Solid Edge part; units mm, degrees
sketch "Sketch1" plane through (0, 0, 0) normal (0, -1, 0) x (1, 0, 0)
  line L0 (40, 40) -> (-40, 40)
  line L1 (-40, 40) -> (-40, -40)
  line L2 (-40, -40) -> (40, -40)
  line L3 (40, -40) -> (40, 40)
  circle A0 centre (0, 0) radius 24
extrude "Extrusionsausprägung_23" add sketch "Sketch1" against normal blind 10
hole "Bohrung_5" at (0, 0, 30) direction (0, 1, 0) diameter 5.5 end up to next
hole "Hole1" at (30, 0, 0) direction (0, 1, 0) diameter 5.5 end up to next
hole "Hole2" at (0, 0, -30) direction (0, 1, 0) diameter 5.5 end up to next
hole "Hole3" at (-30, 0, 0) direction (0, 1, 0) diameter 5.5 end up to next
sketch "Sketch2" plane through (0, 0, 0) normal (0, -1, 0) x (1, 0, 0)
  circle A0 centre (-30, 30) radius 6.35
  circle A1 centre (30, 30) radius 6.35
  circle A2 centre (30, -30) radius 6.35
  circle A3 centre (-30, -30) radius 6.35
extrude "Extrusionsausschnitt_26" cut sketch "Sketch2" against normal blind 274
Design review of the part built by this model. Coordinates are the model's own, in mm. Round coordinates to 2 decimals unless told otherwise and drop trailing zeros. Order: outer loops, then holes, each group sorted by start corner. A loop starts at its lowest first (then second) coordinate and runs counter-clockwise, first axis right, second up. Notation, with made-up numbers: (-21.5, 2) - (21.5, 2) arc R17 ccw to (21.5, 9) - close; hole circle Ø10 at (21, -23.75). An arc over 180 degrees is marked (long way). One line per question, with ' | ' between items.
Item 1: Take a section at C-C, the plane y = 3.25. Give the number of separate pieces and of enclosed holes in the cut face, then the cut area to 3 significant figures.
Checks:
separate pieces: 1 | enclosed holes: 9 | area: 3,990 mm²
Item 2: For P1, Ø6.5, axis at x = 0, z = 30, coming from the -Y side, flat-tipped, find the tip position at first contact; note if it passes through.
Checks:
P1: y = 0
Item 3: Take a section at A-A, the plane x = 0. Write out the cut boundary in (y, z), then the cut area to 3 significant figures.
Checks:
outline: (0, -40) - (10, -40) - (10, -32.75) - (0, -32.75) - close; (0, -27.25) - (10, -27.25) - (10, -24) - (0, -24) - close; (0, 24) - (10, 24) - (10, 27.25) - (0, 27.25) - close; (0, 32.75) - (10, 32.75) - (10, 40) - (0, 40) - close | area: 210 mm²
Item 4: Take a section at D-D, the plane x = -13. Write out the cut boundary in (y, z).
Checks:
outline: (0, -40) - (10, -40) - (10, -20.17) - (0, -20.17) - close; (0, 20.17) - (10, 20.17) - (10, 40) - (0, 40) - close
Item 5: Draft analysis for pull direction X (two halves, no side actions). For faces 1 (the face through (1, 5, 40)), 2 (the face through (-23.977, 4.93, 1.055)), 3 (the face through (-40, 5, 1)), state which applies: +X half, -X half, draft (parallel to the pull), parting line (faces both ways), or undercut.
Checks:
face 1: draft | face 2: undercut | face 3: -X half
Item 6: Wall thickness on line 1 (Z direction, x = 0, y = 6.5); line 2 (Z direction, x = -30, y = 7.5); line 3 (Z direction, x = 34, y = 1.5): over which ranges is each line inside the solid? List them lowest first. Write a range as [from, to].
Checks:
line 1: [-40, -32.75], [-27.25, -24], [24, 27.25], [32.75, 40] | line 2: [-40, -36.35], [-23.65, -2.75], [2.75, 23.65], [36.35, 40] | line 3: [-40, -34.93], [-25.07, 25.07], [34.93, 40]
Item 7: Take a section at B-B, the plane z = -30. Write out the cut boundary in (x, y), then the cut area to 3 significant figures.
Checks:
outline: (-40, 0) - (-36.35, 0) - (-36.35, 10) - (-40, 10) - close; (-23.65, 0) - (-2.75, 0) - (-2.75, 10) - (-23.65, 10) - close; (2.75, 0) - (23.65, 0) - (23.65, 10) - (2.75, 10) - close; (36.35, 0) - (40, 0) - (40, 10) - (36.35, 10) - close | area: 491 mm²
